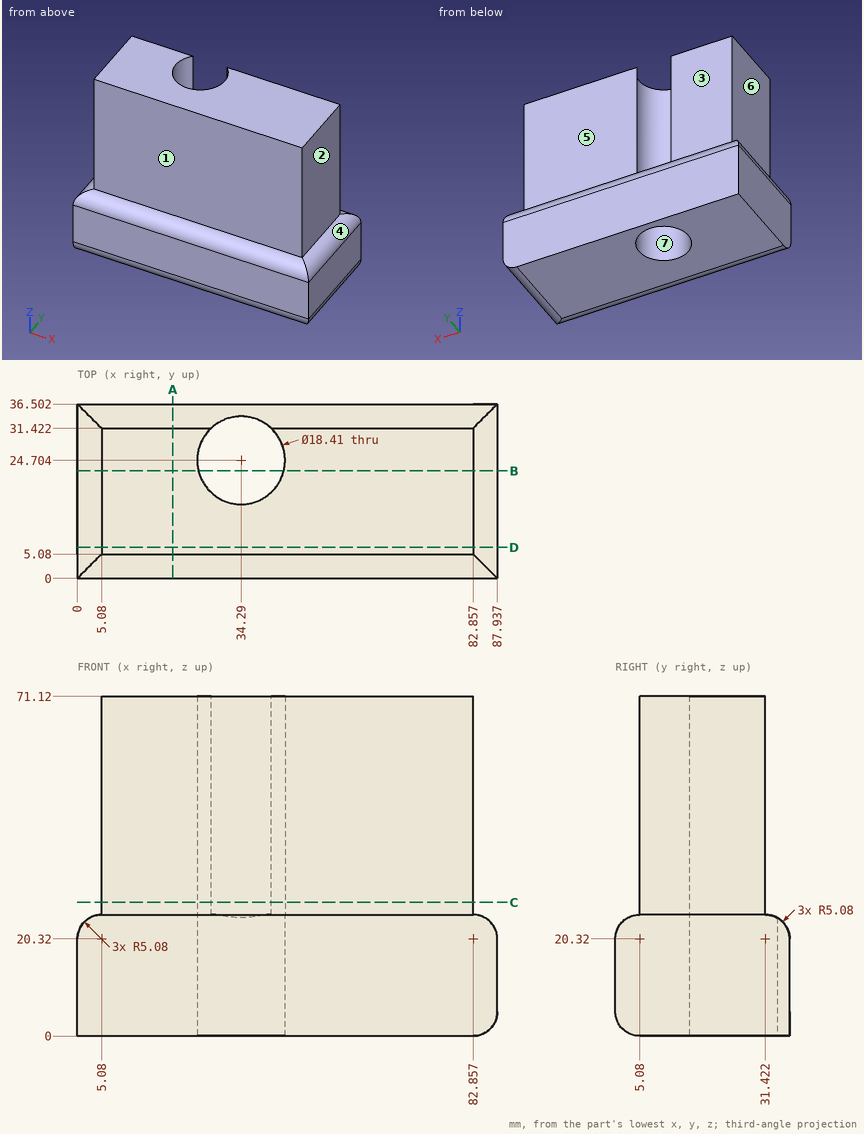
Answer from the drawing. Dimensions are ordinates in mm from the lowest x, y and z of the part. A direction names the side the tool comes from. Coordinates: 2 decimals unless noted, no trailing zeros. Loops run counter-clockwise (first coordinate to the right, second up) from the corner with the lowest first, then second, coordinate; pieces in that order, holes last.
Q1. The part is cut by section C-C on z = 28. Write down the section's boundary in (x, y) (1 decimal), and give its area (3 significant figures).
Q2. The mould has two halves that part along X. Classify the marked faces 4, 5, 6 and 7: +X half, -X half, draft (parallel to the pull), parting line (faces both ways), or undercut.
Q3. Each of these flat-tipped pins is pushed along its axis until it touches: pin 1 Ø5 at (y, z) = (9.5, 40.5) entering from -X; pin 2 Ø11 at (x, y) = (34.29, 24.7) entering from -Z; pin 3 Ø23 at (x, z) = (50.5, 40.5) entering from -Y; pin 4 Ø2 at (y, z) = (6.5, 35) entering from +X. Where does it stop, or does it pass through?
Q4. The part is cut by section D-D on y = 6.5. Write down the section's boundary in (x, z), and give its area (3 significant figures).
Q5. Consider probe 1 along Y at (x, z) = (34, 39); probe 2 along X at (y, z) = (14, 62.5); probe 3 along Y at (x, z) = (80.5, 63). Determine where each line is inside the solid, lowest interval first.
Q6. The part is cut by section A-A on x = 20. Write down the section's boundary in (y, z), and give its area (4 significant figures).
Q7. The part is cut by section B-B on y = 22.5. Write down the section's boundary in (x, z).
Q8. Which of the six approach directions +Z, -Z, +X, -X, +Y, -Y give full straight-line access (tool end or side, diameter ignored) to the marked faces 1, 2 and 3?
Results below:
1. outline: (5.1, 5.1) - (82.9, 5.1) - (82.9, 31.4) - (40.6, 31.4) arc R9.2 cw (long way) to (28, 31.4) - (5.1, 31.4) - close
1. area: 1,800 mm2
2. face 4: +X half
2. face 5: draft
2. face 6: -X half
2. face 7: undercut
3. pin 1: stops at x = 5.08
3. pin 2: passes through
3. pin 3: stops at y = 5.08
3. pin 4: stops at x = 82.86
4. outline: (0, 0) - (82.86, 0) arc R5.08 ccw to (87.94, 5.08) - (87.94, 20.32) arc R5.08 ccw to (82.86, 25.4) - (82.86, 71.12) - (5.08, 71.12) - (5.08, 25.4) arc R5.08 ccw to (0, 20.32) - close
4. area: 5,770 mm2
5. probe 1: y = 5.08 to 15.5
5. probe 2: x = 5.08 to 82.86
5. probe 3: y = 5.08 to 31.42
6. outline: (0, 5.08) arc R5.08 ccw to (5.08, 0) - (36.5, 0) - (36.5, 20.32) arc R5.08 ccw to (31.42, 25.4) - (31.42, 71.12) - (5.08, 71.12) - (5.08, 25.4) arc R5.08 ccw to (0, 20.32) - close
6. area: 2,115 mm2
7. outline: (0, 0) - (25.35, 0) - (25.35, 71.12) - (5.08, 71.12) - (5.08, 25.4) arc R5.08 ccw to (0, 20.32) - close; (43.23, 0) - (82.86, 0) arc R5.08 ccw to (87.94, 5.08) - (87.94, 20.32) arc R5.08 ccw to (82.86, 25.4) - (82.86, 71.12) - (43.23, 71.12) - close
8. face 1: +Z, +X, -X, -Y
8. face 2: +Z, +X, +Y, -Y
8. face 3: +Z, +X, -X, +Y
